from build123d import *

# Parameters (mm, degrees)
BOX002_W          = 22
BOX002_H          = 4.15
BOX002_DEPTH      = 10
CYLINDER002_R     = 15.5
CYLINDER002_DEPTH = 10
CYLINDER001_R     = 21.5
CYLINDER001_DEPTH = 10
BOX001_W          = 200
BOX001_H          = 100
BOX001_DEPTH      = 10
CYLINDER_R        = 21.5
CYLINDER_DEPTH    = 10
BOX_W             = 80
BOX_H             = 80
BOX_DEPTH         = 10


with BuildPart() as cube:
    # Box002 → Box002 (new body)
    with BuildSketch(Plane(origin=(58, 49.36, 0), x_dir=(1, 0, 0), z_dir=(0, 0, 1))):
        with Locations((11, 2.075)):
            Rectangle(BOX002_W, BOX002_H)
    extrude(amount=BOX002_DEPTH)


with BuildPart() as cylinder002:
    # Cylinder002 → Cylinder002 (new body)
    with BuildSketch(Plane(origin=(-25.5, 25.5, 0), x_dir=(1, 0, 0), z_dir=(0, 0, 1))):
        Circle(CYLINDER002_R)
    extrude(amount=CYLINDER002_DEPTH)


with BuildPart() as cylinder001:
    # Cylinder001 → Cylinder001 (new body)
    with BuildSketch(Plane(origin=(38.5, 44.7, 0), x_dir=(1, 0, 0), z_dir=(0, 0, 1))):
        Circle(CYLINDER001_R)
    extrude(amount=CYLINDER001_DEPTH)


with BuildPart() as cut001:
    # Box001 → Box001 (new body)
    with BuildSketch(Plane(origin=(-120, 0, 0), x_dir=(1, 0, 0), z_dir=(0, 0, 1))):
        with Locations((100, 50)):
            Rectangle(BOX001_W, BOX001_H)
    extrude(amount=BOX001_DEPTH)

    # Cut001: cut Cylinder001
    add(cylinder001.part, mode=Mode.SUBTRACT)


with BuildPart() as cylinder:
    # Cylinder → Cylinder (new body)
    with BuildSketch(Plane(origin=(38.5, 44.7, 0), x_dir=(1, 0, 0), z_dir=(0, 0, 1))):
        Circle(CYLINDER_R)
    extrude(amount=CYLINDER_DEPTH)


with BuildPart() as cut003:
    # Box → Box (new body)
    with BuildSketch(Plane.XY):
        with Locations((40, 40)):
            Rectangle(BOX_W, BOX_H)
    extrude(amount=BOX_DEPTH)

    # Cut: cut Cylinder
    add(cylinder.part, mode=Mode.SUBTRACT)

    # Fusion: union Cut001
    add(cut001.part)

    # Cut002: cut Cylinder002
    add(cylinder002.part, mode=Mode.SUBTRACT)

    # Cut003: cut Cube
    add(cube.part, mode=Mode.SUBTRACT)


solid = cut003.part
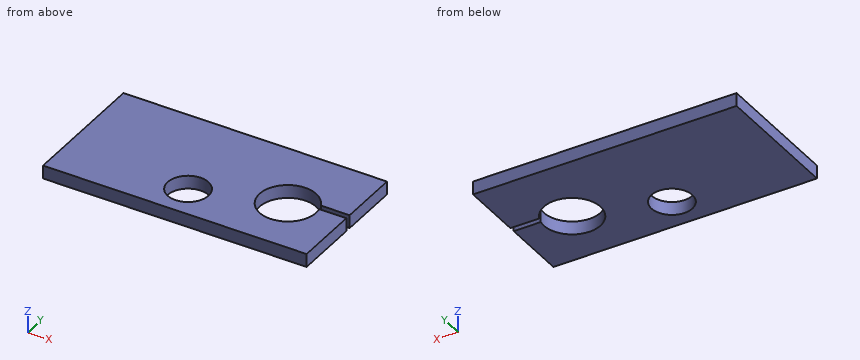
Read the model definition and answer for the solid it produces. Units are mm, in the model's axes. Coordinates: 2 decimals unless noted, no trailing zeros. Write each loop counter-clockwise with the first axis right and the second up, starting at its lowest first coordinate (ties: lowest second). Pieces come first, ordered by that corner, then holes. Notation, with made-up numbers: (46.5, 27.25) -> (73.5, 27.25) arc R8 cw to (73.5, 34.25) -> close; hole circle Ø1 at (69.5, -9). An arc over 180 degrees is marked (long way). Return JSON: item names as keys, results as strings.
(1) The part is cut by section B-B on z = 7.5. Give the vertices of the cut face in (x, y), then the cut area to 3 significant figures.
Answers below:
{"outline": "(-120, 0) -> (80, 0) -> (80, 49.36) -> (59.49, 49.36) arc R21.5 cw (long way) to (58.11, 53.51) -> (80, 53.51) -> (80, 100) -> (-120, 100) -> close; hole circle Ø31 at (-25.5, 25.5)", "area": "17,700 mm^2"}
(2) Consider line 1 along Y through (x, z) = (38.5, 3.25); line 2 along Y through (x, z) = (-25.5, 7.5); line 3 along X through (y, z) = (44.7, 6.5). Determine where each line is inside the solid, lowest interval first. Write a range as from..to.
Answers below:
{"line 1": "0..23.2, 66.2..100", "line 2": "0..10, 41..100", "line 3": "-120..17, 60..80"}
(3) The part is cut by section A-A on x = -25.5. Give the vertices of the cut face in (y, z).
Answers below:
{"outline": "(0, 0) -> (10, 0) -> (10, 10) -> (0, 10) -> close; (41, 0) -> (100, 0) -> (100, 10) -> (41, 10) -> close"}
(4) The part is cut by section D-D on y = 25.5. Give the vertices of the cut face in (x, z), then the cut area to 3 significant figures.
Answers below:
{"outline": "(-120, 0) -> (-41, 0) -> (-41, 10) -> (-120, 10) -> close; (-10, 0) -> (28.82, 0) -> (28.82, 10) -> (-10, 10) -> close; (48.18, 0) -> (80, 0) -> (80, 10) -> (48.18, 10) -> close", "area": "1,500 mm^2"}
(5) The part is cut by section C-C on y = 44.7. Give the vertices of the cut face in (x, z), then the cut area to 3 significant figures.
Answers below:
{"outline": "(-120, 0) -> (17, 0) -> (17, 10) -> (-120, 10) -> close; (60, 0) -> (80, 0) -> (80, 10) -> (60, 10) -> close", "area": "1,570 mm^2"}
